Source: CAD feature listing. Evaluate the final solid. Frame: model axes, mm. Round coordinates to 2 decimals unless told otherwise and drop trailing zeros. Write item = value, one per line. Start each with the question number.
(1) Ray query, line 1 (X direction, y = 7, z = 231.5); line 2 (Y direction, x = -15, z = 115.5); line 3 (X direction, y = 6.25, z = 405.5). Return the intervals inside material, ascending.
(2) Cut plane A-A on z = 37.5. Give the number of separate pieces and of enclosed holes in the cut face, then the cut area to 3 significant figures.
(3) Contact query for flat-ended pins moving along their axis: pin 1 Ø1.7 at (x, z) = (10.5, 245) entering from +Y; pin 2 Ø0.8 at (x, z) = (6, 255.5) entering from -Y; pin 3 Ø2 at (y, z) = (0.5, 148) entering from +X. Output: stop coordinate, or through.
Autodesk Inventor part; units mm, degrees
ref_plane "Start Plane" through (0, 0, 0) normal (0, 0, 1) x (1, 0, 0)
ref_plane "End Plane" through (0, 0, 10) normal (0, 0, 1) x (1, 0, 0)
ref_plane "YZ Plane" through (0, 0, 0) normal (1, 0, 0) x (0, 1, 0)
ref_plane "Start Plane" through (0, 0, 0) normal (0, 0, 1) x (1, 0, 0)
ref_plane "End Plane" through (0, 0, 10) normal (0, 0, 1) x (1, 0, 0)
sketch "Sketch3" plane through (0, 0, 0) normal (0, 0, 1) x (1, 0, 0)
  line L0 (0, 0) -> (0, 10) construction
  line L1 (-10, 10) -> (-10, 0) construction
  line L2 (0, 0) -> (-10, 0) construction
  circle A0 centre (-10, 0) radius 2.1
  line L3 (-13.9007, 3.9007) -> (-6.0993, 3.9007) construction
  line L4 (-6.0993, 3.9007) -> (-6.0993, -3.9007) construction
  line L5 (-6.0993, -3.9007) -> (-13.9007, -3.9007) construction
  line L6 (-13.9007, -3.9007) -> (-13.9007, 3.9007) construction
  line L7 (-13.9007, 3.9007) -> (-6.0993, -3.9007) construction
  line L8 (-6.0993, 3.9007) -> (-13.9007, -3.9007) construction
  line L9 (-13.9007, -2.84) -> (-12.84, -3.9007) construction
  line L10 (-13.9007, -2.84) -> (-12.4007, -2.84) construction
  line L11 (-12.84, -3.9007) -> (-15.4993, -6.56)
  line L12 (-15.4993, -6.56) -> (-15.4993, -8.2)
  line L13 (-15.4993, -8.2) -> (-12.84, -8.2)
  line L14 (-12.84, -8.2) -> (-14.64, -10)
  line L15 (-7.16, -3.9007) -> (-4.5007, -6.56)
  line L16 (-4.5007, -6.56) -> (-4.5007, -8.2)
  line L17 (-4.5007, -8.2) -> (-7.16, -8.2)
  line L18 (-7.16, -8.2) -> (-5.36, -10)
  line L19 (-12.84, -3.9007) -> (-7.16, -3.9007)
  line L20 (-12.84, 3.9007) -> (-13.9007, 2.84) construction
  line L21 (-12.84, 3.9007) -> (-12.84, 2.4007) construction
  line L22 (-13.9007, 2.84) -> (-16.56, 5.4993)
  line L23 (-16.56, 5.4993) -> (-18.2, 5.4993)
  line L24 (-18.2, 5.4993) -> (-18.2, 2.84)
  line L25 (-18.2, 2.84) -> (-20, 4.64)
  line L26 (-18.2, -2.84) -> (-20, -4.64)
  line L27 (-18.2, -5.4993) -> (-18.2, -2.84)
  line L28 (-16.56, -5.4993) -> (-18.2, -5.4993)
  line L29 (-13.9007, -2.84) -> (-16.56, -5.4993)
  line L30 (-13.9007, 2.84) -> (-13.9007, -2.84)
  line L31 (-6.0993, 2.84) -> (-7.16, 3.9007) construction
  line L32 (-6.0993, 2.84) -> (-7.5993, 2.84) construction
  line L33 (-7.16, 3.9007) -> (-4.5007, 6.56)
  line L34 (-4.5007, 6.56) -> (-4.5007, 8.2)
  line L35 (-4.5007, 8.2) -> (-7.16, 8.2)
  line L36 (-7.16, 8.2) -> (-5.36, 10)
  line L37 (-12.84, 8.2) -> (-14.64, 10)
  line L38 (-15.4993, 8.2) -> (-12.84, 8.2)
  line L39 (-15.4993, 6.56) -> (-15.4993, 8.2)
  line L40 (-12.84, 3.9007) -> (-15.4993, 6.56)
  line L41 (-7.16, 3.9007) -> (-12.84, 3.9007)
  line L42 (-6.0993, 2.84) -> (-2.6993, 6.24)
  line L43 (-2.6993, 6.24) -> (-2.6993, 8.2)
  line L44 (-4.5007, 8.2) -> (0, 8.2) construction
  line L45 (-6.0993, -2.84) -> (-2.6993, -6.24)
  line L46 (-2.6993, -6.24) -> (-2.6993, -8.2)
  line L47 (10, 10) -> (10, 0) construction
  circle A1 centre (10, 0) radius 2.1
  line L48 (13.9007, 3.9007) -> (6.0993, -3.9007) construction
  line L49 (13.9007, -2.84) -> (12.84, -3.9007) construction
  line L50 (12.84, -3.9007) -> (15.4993, -6.56)
  line L51 (15.4993, -6.56) -> (15.4993, -8.2)
  line L52 (15.4993, -8.2) -> (12.84, -8.2)
  line L53 (12.84, -8.2) -> (14.64, -10)
  line L54 (7.16, -8.2) -> (5.36, -10)
  line L55 (4.5007, -8.2) -> (7.16, -8.2)
  line L56 (4.5007, -6.56) -> (4.5007, -8.2)
  line L57 (7.16, -3.9007) -> (4.5007, -6.56)
  line L58 (12.84, -3.9007) -> (7.16, -3.9007)
  line L59 (13.9007, 2.84) -> (13.9007, -2.84)
  line L60 (13.9007, 2.84) -> (16.56, 5.4993)
  line L61 (16.56, 5.4993) -> (18.2, 5.4993)
  line L62 (18.2, 5.4993) -> (18.2, 2.84)
  line L63 (18.2, 2.84) -> (20, 4.64)
  line L64 (18.2, -5.4993) -> (18.2, -2.84)
  line L65 (18.2, -2.84) -> (20, -4.64)
  line L66 (16.56, -5.4993) -> (18.2, -5.4993)
  line L67 (13.9007, -2.84) -> (16.56, -5.4993)
  line L68 (7.16, 3.9007) -> (12.84, 3.9007)
  line L69 (7.16, 3.9007) -> (4.5007, 6.56)
  line L70 (4.5007, 6.56) -> (4.5007, 8.2)
  line L71 (4.5007, 8.2) -> (7.16, 8.2)
  line L72 (7.16, 8.2) -> (5.36, 10)
  line L73 (15.4993, 8.2) -> (12.84, 8.2)
  line L74 (12.84, 8.2) -> (14.64, 10)
  line L75 (15.4993, 6.56) -> (15.4993, 8.2)
  line L76 (12.84, 3.9007) -> (15.4993, 6.56)
  line L77 (6.0993, 2.84) -> (2.6993, 6.24)
  line L78 (2.6993, 6.24) -> (2.6993, 8.2)
  line L79 (6.0993, -2.84) -> (2.6993, -6.24)
  line L80 (2.6993, -6.24) -> (2.6993, -8.2)
  line L81 (-14.64, -10) -> (-18.2, -10)
  line L82 (-20, -8.2) -> (-20, -4.64)
  line L83 (-20, 4.64) -> (-20, 8.2)
  line L84 (-18.2, 10) -> (-14.64, 10)
  line L85 (18.2, -10) -> (14.64, -10)
  line L86 (5.36, -10) -> (-5.36, -10)
  line L87 (-5.36, 10) -> (5.36, 10)
  line L88 (14.64, 10) -> (18.2, 10)
  line L89 (20, 8.2) -> (20, 4.64)
  line L90 (20, -4.64) -> (20, -8.2)
  line L91 (-2.6993, -8.2) -> (2.6993, -8.2)
  line L92 (-2.6993, 8.2) -> (2.6993, 8.2)
  line L93 (-6.0993, 2.84) -> (-6.0993, -2.84)
  line L94 (6.0993, 2.84) -> (6.0993, -2.84)
  arc A2 (-20, -8.2) -> (-18.2, -10) centre (-18.2, -8.2) ccw
  arc A3 (-18.2, 10) -> (-20, 8.2) centre (-18.2, 8.2) ccw
  arc A4 (18.2, -10) -> (20, -8.2) centre (18.2, -8.2) ccw
  arc A5 (20, 8.2) -> (18.2, 10) centre (18.2, 8.2) ccw
  point P0 (-13.9007, -3.9007)
  point P1 (-13.9007, 3.9007)
  point P2 (-13.9007, 3.9007)
  point P3 (-6.0993, 3.9007)
  point P4 (6.0993, 3.9007)
  point P5 (13.9007, -3.9007)
  point P6 (12.4007, -2.84)
  point P7 (13.9007, -3.9007)
  point P8 (13.9007, 3.9007)
  point P9 (12.84, 3.9007)
  point P10 (12.84, 2.4007)
  point P11 (13.9007, 3.9007)
  point P12 (6.0993, 3.9007)
  point P13 (7.5993, 2.84)
  point P14 (-20, 10)
  point P15 (20, -10)
  point P16 (20, 10)
  point P17 (-20, -10)
  dimension "d26" = 10
  dimension "d27" = 10
  dimension "d28" = 4.2
  dimension "d29" = 1.5
  dimension "d30" = 45
  dimension "d32" = 45
  dimension "d33" = 1.64
  dimension "d34" = 1.8
  dimension "d35" = 10
  dimension "d36" = 5.68
  dimension "d39" = 180
  dimension "d41" = 1.96
  dimension "d42" = 5.68
  dimension "d45" = 1.8
extrude "Body" add sketch "Sketch3" along normal blind 500
sketch "Sketch4" plane through (0, 0, 0) normal (0, 0, 1) x (1, 0, 0)
  line L0 (0, 0) -> (10, 0)
ref_plane "Work Plane3" through (0, 0, 0) normal (0, -1, 0) x (1, 0, 0)
sketch "Sketch5" plane through (0, 0, 0) normal (0, -1, 0) x (1, 0, 0)
  line L0 (-2, 0) -> (12, 0)
  line L1 (-2, 10) -> (12, 10)
  dimension "d51" = 10
equation "\"d42\" = d36"
equation "\"G_OFFSET_START\" = 0"
equation "\"G_OFFSET_END\" = 0"
equation "\"G_L\" = d51"
properties part number "vslot 20 x 40" material "Aluminum 6061"
Evaluation:
q1.line_1 = -20 to -15.5, -4.5 to -2.7, 2.7 to 4.5, 15.5 to 20
q1.line_2 = -10 to -8.2, -6.06 to -3.94, 3.94 to 6.06, 8.2 to 10
q1.line_3 = -20 to -15.19, -4.81 to -2.7, 2.7 to 4.81, 15.19 to 20
q2.separate_pieces = 1
q2.enclosed_holes = 3
q2.area = 297 mm^2
q3.pin_1 = 3.9
q3.pin_2 = -9.76
q3.pin_3 = 13.9
